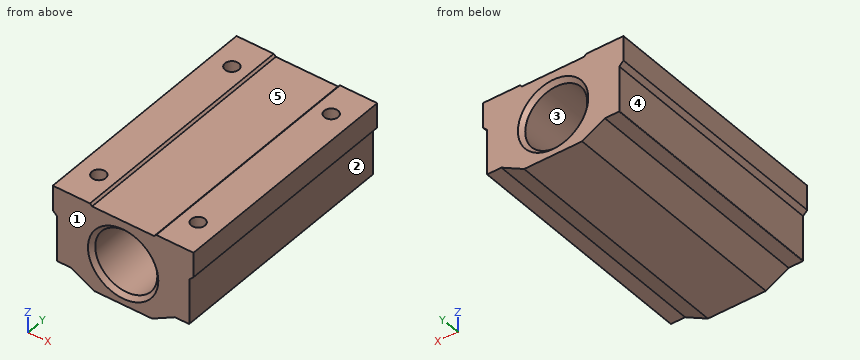
Autodesk Fusion 360 part; units mm, degrees
sketch "Sketch1" plane through (0, 0, 0) normal (0, 1, 0) x (1, 0, 0)
  circle A0 centre (0, 0) radius 7.5
  line L0 (-17, -11) -> (17, -11)
  line L1 (17, -11) -> (17, -5)
  line L2 (17, -5) -> (16, -4)
  line L3 (16, -4) -> (16, 7)
  line L4 (16, 7) -> (12.5, 7)
  line L5 (12.5, 7) -> (7, 10)
  line L6 (-17, -11) -> (-17, -5)
  line L7 (-17, -5) -> (-16, -4)
  line L8 (-16, -4) -> (-16, 7)
  line L9 (-16, 7) -> (-12.5, 7)
  line L10 (-12.5, 7) -> (-7, 10)
  line L11 (-7, 10) -> (7, 10)
  dimension "d1" = 15
  dimension "d2" = 34
  dimension "d3" = 14
  dimension "d4" = 21
extrude "Extrude1" add sketch "Sketch1" along normal mid plane 58
sketch "Sketch2" plane through (0, 0, 11) normal (0, 0, 1) x (-1, 0, 0)
  line L0 (-17, 29) -> (-17, -29)
  line L1 (-17, -29) -> (17, -29)
  line L2 (17, -29) -> (17, 29)
  line L3 (17, 29) -> (-17, 29)
  line L4 (0, -21) -> (0, 21) construction
  line L5 (17, 0) -> (-17, 0) construction
  line L6 (-12, -21) -> (12, -21) construction
  line L7 (12, 21) -> (-12, 21) construction
  circle A0 centre (-12, -21) radius 2
  circle A1 centre (-12, 21) radius 2
  circle A2 centre (12, 21) radius 2
  circle A3 centre (12, -21) radius 2
  line L8 (8, -29) -> (8, 29)
  line L9 (-10, -21) -> (-8, -21)
  line L10 (-8, -29) -> (-8, 29)
  dimension "d7" = 42
  dimension "d8" = 24
  dimension "d13" = 16
hole "Hole1" at (12, 21, 11) at (-12, 21, 11) at (-12, -21, 11) at (12, -21, 11) direction (0, 0, -1) diameter 3.332 depth 8 tip angle 118
chamfer "Chamfer1" distance 1 angle 45 2 edges at (-6.9925, -29, 2.7121) (-6.9925, 29, -2.7121)
extrude "Extrude2" cut sketch "Sketch2" against normal blind 0.5 contours L1 L3 L8 L10
chamfer "Chamfer2" distance 0.5 angle 45 2 edges at (-8, 0, 10.5) (8, 0, 10.5)
fillet "Fillet1" radius 0.1 2 edges at (16, 0, -7) (-16, 0, -7)
Could you check a few things on this model? Use its own coordinates, in mm. Face numbers are marked on the shaded views. A direction names the side the tool comes from. Coordinates: 2 decimals unless noted, no trailing zeros. Loops run counter-clockwise (first coordinate to the right, second up) from the corner with the lowest first, then second, coordinate; pieces in that order, holes last.
1) Will these pins go through, and if not, where does the flat tip stop? pin 1 Ø2.5 at (x, y) = (12, 21) entering from +Z; pin 2 Ø2.5 at (x, y) = (13.5, 10.5) entering from -Z; pin 3 Ø7.5 at (x, y) = (-3.5, -12.5) entering from +Z.
Reported:
pin 1: stops at z = 2.75
pin 2: stops at z = -7.14
pin 3: stops at z = 10.5
2) Please list where these lines run through material, in increasing order: line 1 along Y through (x, z) = (-12, 7.25); line 2 along X through (y, z) = (21, 8); line 3 along Z through (x, y) = (0, 10).
Reported:
line 1: y = -29 to -22.67, -19.33 to 19.33, 22.67 to 29
line 2: x = -17 to -13.67, -10.33 to 10.33, 13.67 to 17
line 3: z = -10 to -7.5, 7.5 to 10.5
3) Thinking about a two-plate mould opening in Z: for the marked faces 3, 4 and 5, which applies, released by +Z, released by -Z, zero draft, split by the parting line, or undercut?
Reported:
face 3: undercut
face 4: zero draft
face 5: released by +Z
4) Imagine slicing it at A-A (z = 0). List the corners of the cut face in (x, y) for me, and give its area (3 significant figures).
Reported:
outline: (-16, -29) - (-8.5, -29) - (-7.5, -28) - (-7.5, 28) - (-8.5, 29) - (-16, 29) - close; (7.5, -28) - (8.5, -29) - (16, -29) - (16, 29) - (8.5, 29) - (7.5, 28) - close
area: 984 mm2
5) Which directions (+Z, -Z, +X, -X, +Y, -Y) give clear straight access to the entire face, cutting with the end or side of a thin tool? Please do the marked faces 1 and 2.
Reported:
face 1: +Z, -Z, +X, -X, -Y
face 2: -Z, +X, +Y, -Y
6) Imagine slicing it at D-D (z = 9.5). List the corners of the cut face in (x, y) for me, and give its area (3 significant figures).
Reported:
outline: (-17, -29) - (17, -29) - (17, 29) - (-17, 29) - close; hole circle Ø3.33 at (-12, -21); hole circle Ø3.33 at (-12, 21); hole circle Ø3.33 at (12, -21); hole circle Ø3.33 at (12, 21)
area: 1,940 mm2
7) Imagine slicing it at C-C (x = 0). List the corners of the cut face in (y, z) for me.
Reported:
outline: (-29, -10) - (29, -10) - (29, -8.5) - (28, -7.5) - (-28, -7.5) - (-29, -8.5) - close; (-29, 8.5) - (-28, 7.5) - (28, 7.5) - (29, 8.5) - (29, 10.5) - (-29, 10.5) - close
